from build123d import *

# Parameters (mm, degrees)
SKETCH001_W         = 1
SKETCH001_H         = 2
LINEARPATTERN_COUNT = 5
LINEARPATTERN_PITCH = 24


with BuildPart() as part:
    # Sketch → Revolution (revolve)
    with BuildSketch(Plane.XY):
        with BuildLine():
            ThreePointArc((0, 0), (-2.911842, 7.836159), (-10.234231, 11.869375))
            Line((-10.234231, 11.869375), (-38, 16))
            Line((-38, 16), (-138, 16))
            ThreePointArc((-138, 16), (-149.313709, 11.313708), (-154, 0))
            Line((-153, 0), (-154, 0))
            ThreePointArc((-138, 15), (-148.606602, 10.606602), (-153, 0))
            Line((-138, 15), (-38, 15))
            Line((-38, 15), (-10.381764, 10.880318))
            ThreePointArc((-1, 0), (-3.669316, 7.183293), (-10.381764, 10.880318))
            Line((-1, 0), (0, 0))
        make_face()
    revolve(axis=Axis((0, 0, 0), (1, 0, 0)))

    # Sketch001 (on DatumPlane) → Revolution001 (revolve)
    with BuildSketch(Plane.XY):
        with Locations((-137.5, -14)):
            Rectangle(SKETCH001_W, SKETCH001_H)
    revolution001 = revolve(axis=Axis((0, 0, 0), (1, 0, 0)))

    # LinearPattern: Revolution001 ×5
    with Locations(*[(i * LINEARPATTERN_PITCH, 0, 0) for i in range(1, LINEARPATTERN_COUNT)]):
        add(revolution001)

    # Sketch002 (on DatumPlane) → Revolution002 (revolve)
    with BuildSketch(Plane.XY):
        Polygon((-24.1532, -12.934538), (-25.142257, -13.082071), (-25.437323, -11.103957), (-24.448266, -10.956424), align=None)
    revolve(axis=Axis((0, 0, 0), (1, 0, 0)))


solid = part.part
For this review, take the finished solid that the model builds, in its own axes (mm). Give positions to 0.01 mm unless a question says otherwise; leave off trailing zeros. Loops run counter-clockwise (first coordinate to the right, second up) from the corner with the lowest first, then second, coordinate; pieces in that order, holes last.
Item 1: Take a section at B-B, the plane x = -33. State the section outline as (y, z) points.
Item 2: Draft analysis for pull direction Y (two halves, no side actions). For faces 1 (the flat face through (-41, 0.1, -13.4)), 2 (the conical face through (-21.226, -2.928, -13.184)), state which applies: +Y half, -Y half, draft (parallel to the pull), parting line (faces both ways), or undercut.
Item 3: Take a section at A-A, the plane x = -63. State the section outline as (y, z) points, and give its area (3 significant figures).
Item 4: Insertion check: pin 1 (1 mm diameter, centred on y = -4, z = 8.5, fed in from +X); pin 2 (4 mm diameter, centred on x = -57, z = -6, fed in from -Y); pin 3 (1 mm diameter, centred on x = -104, y = 5, fed in from -Z); pin 4 (15 mm diameter, centred on y = -6, z = -1.5, fed in from -X). Each pin has a flat end and moves straight along its axis. Give the tip position at first contact, or say it passes through.
Item 5: For line 1 along Z through (x, y) = (-55, 0); line 2 along Z through (x, y) = (-89.55, 0); line 3 along Y through (x, z) = (-91, 6), list the stretches that pass through material, from the lowest coordinate up.
Calculated:
1. outline: circle Ø30.51 at (0, 0); hole circle Ø28.51 at (0, 0)
2. face 1: undercut
2. face 2: parting line
3. outline: circle Ø32 at (0, 0); hole circle Ø30 at (0, 0)
3. area: 97.4 mm2
4. pin 1: stops at x = -3.94
4. pin 2: stops at y = -15.49
4. pin 3: stops at z = -15.35
4. pin 4: stops at x = -154
5. line 1: z = -16 to -15, 15 to 16
5. line 2: z = -16 to -13, 13 to 16
5. line 3: y = -14.83 to -13.75, 13.75 to 14.83
